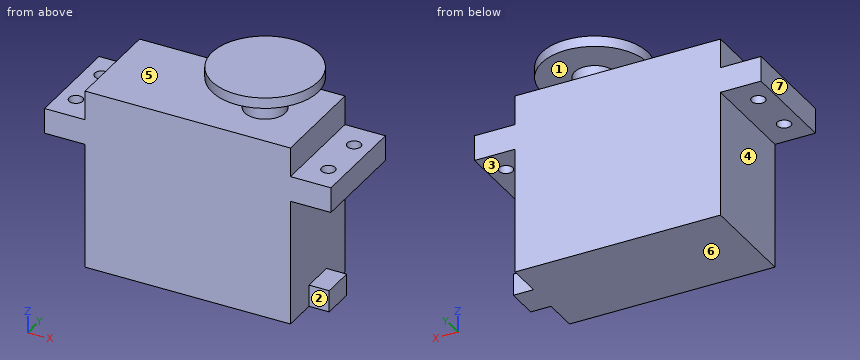
```python
from build123d import *

# Parameters (mm, degrees)
F0_W      = 40.6
F0_H      = 20
F1_DEPTH  = 35.7
F2_W      = 8
F2_H      = 5
F3_DEPTH  = 20
F4_R      = 4
F5_DEPTH  = 6.1
F6_R      = 10.5
F7_DEPTH  = 2.1
F8_W      = 6.4
F8_H      = 4.3
F9_DEPTH  = 4
F10_R     = 1.35
F11_DEPTH = 5


with BuildPart() as f1:
    # F0 (on Top) → F1 (new body)
    with BuildSketch(Plane.XY):
        with Locations((20.3, 10)):
            Rectangle(F0_W, F0_H)
    extrude(amount=F1_DEPTH)

    # F2 (on face) → F3 (join, through all)
    with BuildSketch(Plane.XZ):
        with Locations((44.6, 27.4)):
            Rectangle(F2_W, F2_H)
        with Locations((-4, 27.4)):
            Rectangle(F2_W, F2_H)
    extrude(amount=-F3_DEPTH)

    # F4 (on face) → F5 (join)
    with BuildSketch(Plane.XY.offset(35.7)):
        with Locations((30.2, 10)):
            Circle(F4_R)
    extrude(amount=F5_DEPTH)

    # F6 (on face) → F7 (join)
    with BuildSketch(Plane.XY.offset(41.8)):
        with Locations((30.2, 10)):
            Circle(F6_R)
    extrude(amount=F7_DEPTH)

    # F8 (on face) → F9 (join)
    with BuildSketch(Plane.YZ.offset(40.6)):
        with Locations((10, 2.15)):
            Rectangle(F8_W, F8_H)
    extrude(amount=F9_DEPTH)

    # F10 (on face) → F11 (cut, through all)
    with BuildSketch(Plane.XY.offset(29.9)):
        with Locations((-4.65, 14.7)):
            Circle(F10_R)
        with Locations((-4.65, 5.3)):
            Circle(F10_R)
        with Locations((45.25, 14.7)):
            Circle(F10_R)
        with Locations((45.25, 5.3)):
            Circle(F10_R)
    extrude(amount=-F11_DEPTH, mode=Mode.SUBTRACT)


solid = f1.part
```
The listing builds one solid part. Answer for the finished solid, in the listing's coordinates (mm). Face numbers are marked on the shaded views. A direction names the side the tool comes from. Coordinates: 2 decimals unless noted, no trailing zeros. Loops run counter-clockwise (first coordinate to the right, second up) from the corner with the lowest first, then second, coordinate; pieces in that order, holes last. Notation, with made-up numbers: (29, 59.5) -> (49, 59.5) arc R13 cw to (49, 69.5) -> close; hole circle Ø3 at (53.25, 79.25). An arc over 180 degrees is marked (long way). Use one line per item in the form item = value. Start each with the question number.
Item 1: The part is cut by section D-D on x = 30.2. Determine the outline of the cut face in (y, z), then the cut area to 3 significant figures.
Item 2: The part is cut by section C-C on y = 10. Determine the outline of the cut face in (x, z).
Item 3: The part is cut by section B-B on y = 14.7. Determine the outline of the cut face in (x, z).
Item 4: A tool of negligible diameter and unlimited length cuts with its end or side. For the marked faces 1, 2, 3 and 4, from which of +Z, -Z, +X, -X, +Y, -Y can it reach the whole face along a straight path? Write none if from no direction.
Item 5: Consider L1, parallel to Y at x = -4.65, z = 27.55; L2, parallel to Z at x = 37.5, y = 9; L3, parallel to Y at x = -4, z = 26. Determine where each line is inside the solid, lowest interval first. Write a range as [from, to].
Item 6: The part is cut by section A-A on x = -4.65. Determine the outline of the cut face in (y, z), then the cut area to 3 significant figures.
Item 7: The mould has two halves that part along Z. Classify the marked faces 5, 6 and 7: released by +Z, released by -Z, zero draft, split by the parting line, or undercut.
Item 8: Flat-ended cylindrical pins translate along their axes: pin 1 Ø3 at (x, y) = (45.25, 5.3) entering from +Z; pin 2 Ø9 at (x, y) = (-3, 8) entering from -Z; pin 3 Ø1.7 at (y, z) = (7, 33.5) entering from +X; pin 4 Ø2 at (x, z) = (19.5, 16.5) entering from +Y. Find the tip coordinate at first contact, or state that the pin passes through.
Answer key:
q1.outline = (-0.5, 41.8) -> (6, 41.8) -> (6, 35.7) -> (0, 35.7) -> (0, 0) -> (20, 0) -> (20, 35.7) -> (14, 35.7) -> (14, 41.8) -> (20.5, 41.8) -> (20.5, 43.9) -> (-0.5, 43.9) -> close
q1.area = 807 mm2
q2.outline = (-8, 24.9) -> (0, 24.9) -> (0, 0) -> (44.6, 0) -> (44.6, 4.3) -> (40.6, 4.3) -> (40.6, 24.9) -> (48.6, 24.9) -> (48.6, 29.9) -> (40.6, 29.9) -> (40.6, 35.7) -> (34.2, 35.7) -> (34.2, 41.8) -> (40.7, 41.8) -> (40.7, 43.9) -> (19.7, 43.9) -> (19.7, 41.8) -> (26.2, 41.8) -> (26.2, 35.7) -> (0, 35.7) -> (0, 29.9) -> (-8, 29.9) -> close
q3.outline = (-8, 24.9) -> (-6, 24.9) -> (-6, 29.9) -> (-8, 29.9) -> close; (-3.3, 24.9) -> (0, 24.9) -> (0, 0) -> (40.6, 0) -> (40.6, 24.9) -> (43.9, 24.9) -> (43.9, 29.9) -> (40.6, 29.9) -> (40.6, 35.7) -> (0, 35.7) -> (0, 29.9) -> (-3.3, 29.9) -> close; (20.81, 41.8) -> (39.59, 41.8) -> (39.59, 43.9) -> (20.81, 43.9) -> close; (46.6, 24.9) -> (48.6, 24.9) -> (48.6, 29.9) -> (46.6, 29.9) -> close
q4.face_1 = none
q4.face_2 = -Z, +X, -Y
q4.face_3 = +X, +Y, -Y
q4.face_4 = -Z, -X, +Y, -Y
q5.L1 = [0, 3.95], [6.65, 13.35], [16.05, 20]
q5.L2 = [0, 35.7], [41.8, 43.9]
q5.L3 = [0, 4.12], [6.48, 13.52], [15.88, 20]
q6.outline = (0, 24.9) -> (3.95, 24.9) -> (3.95, 29.9) -> (0, 29.9) -> close; (6.65, 24.9) -> (13.35, 24.9) -> (13.35, 29.9) -> (6.65, 29.9) -> close; (16.05, 24.9) -> (20, 24.9) -> (20, 29.9) -> (16.05, 29.9) -> close
q6.area = 73.0 mm2
q7.face_5 = undercut
q7.face_6 = released by -Z
q7.face_7 = zero draft
q8.pin_1 = 29.9
q8.pin_2 = 0
q8.pin_3 = 40.6
q8.pin_4 = 20
